Build history of the part. All positions in model axes, mm. Coordinates: 2 decimals unless noted, no trailing zeros. Order: outer loops, then holes, each group sorted by start corner. A loop starts at its lowest first (then second) coordinate and runs counter-clockwise, first axis right, second up. Notation, with made-up numbers: (60.5, 24.25) - (107.5, 24.25) arc R6 cw to (107.5, 35.25) - close; hole circle Ø9 at (73.25, 67). An arc over 180 degrees is marked (long way). One line per item, written item: value.
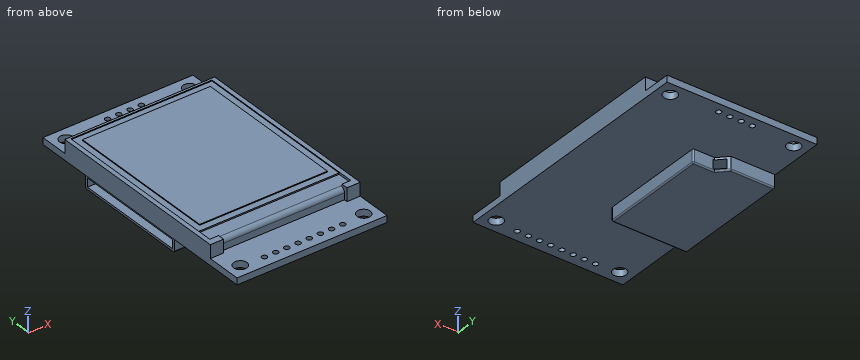
Autodesk Fusion 360 part; units mm, degrees
sketch "Sketch1" plane through (0, 0, 0) normal (0, 0, 1) x (1, 0, 0)
  line L0 (0, 0) -> (34, 0)
  line L1 (34, 0) -> (34, 58)
  line L2 (34, 58) -> (0, 58)
  line L3 (0, 58) -> (0, 0)
  circle A0 centre (3, 3) radius 1.5
  circle A1 centre (31, 3) radius 1.5
  circle A2 centre (3, 55) radius 1.5
  circle A3 centre (31, 55) radius 1.5
  dimension "d1" = 34
  dimension "d2" = 58
  dimension "d3" = 3
  dimension "d4" = 3
  dimension "d5" = 3
  dimension "d6" = 3
  dimension "d7" = 3
  dimension "d8" = 3
  dimension "d9" = 3
  dimension "d10" = 3
  dimension "d11" = 3
  dimension "d12" = 3
  dimension "d13" = 3
  dimension "d14" = 3
extrude "Extrude1" add sketch "Sketch1" along normal blind 1.5
sketch "Sketch2" plane through (0, 0, 1.5) normal (0, 0, 1) x (-1, 0, 0)
  circle A0 centre (-31, -3) radius 1.5
  circle A1 centre (-3, -55) radius 1.5
  circle A2 centre (-3, -3) radius 1.5
  circle A3 centre (-31, -55) radius 1.5
  line L0 (0, -58) -> (0, 0)
  line L1 (0, 0) -> (-34, 0)
  line L2 (-34, 0) -> (-34, -58)
  line L3 (-34, -58) -> (0, -58)
  line L4 (0, -8) -> (-34, -8)
  line L5 (-34, -8) -> (-34, -51.5)
  line L6 (-34, -51.5) -> (0, -51.5)
  line L7 (0, -51.5) -> (0, -8)
  dimension "d17" = 43.5
  dimension "d18" = 34
  dimension "d19" = 8
extrude "Extrude2" add sketch "Sketch2" along normal blind 3 contours L0 L2 L4 L5 L6 L7
sketch "Sketch3" plane through (0, 0, 4.5) normal (0, 0, 1) x (-1, 0, 0)
  line L0 (0, -51.5) -> (0, -8)
  line L1 (0, -8) -> (-34, -8)
  line L2 (-34, -8) -> (-34, -51.5)
  line L3 (-34, -51.5) -> (0, -51.5)
  line L4 (-1, -13) -> (-33, -13)
  line L5 (-33, -13) -> (-33, -51)
  line L6 (-33, -51) -> (-1, -51)
  line L7 (-1, -51) -> (-1, -13)
  line L8 (-3, -13) -> (-31, -13)
  line L9 (-31, -13) -> (-31, -8)
  line L10 (-31, -8) -> (-3, -8)
  line L11 (-3, -8) -> (-3, -13)
  line L12 (-3, -9.5) -> (-1, -9.5)
  line L13 (-1, -9.5) -> (-1, -13)
  line L14 (-1, -13) -> (-3, -13)
  line L15 (-3, -13) -> (-3, -9.5)
  line L16 (-31, -9.5) -> (-33, -9.5)
  line L17 (-33, -9.5) -> (-33, -13)
  line L18 (-33, -13) -> (-31, -13)
  line L19 (-31, -13) -> (-31, -9.5)
  dimension "d22" = 5
  dimension "d23" = 0.5
  dimension "d24" = 1
  dimension "d25" = 1
  dimension "d38" = 28
  dimension "d39" = 3
  dimension "d42" = 1.5
  dimension "d43" = 1.5
extrude "Extrude6" cut sketch "Sketch3" against normal blind 3 contours L4 L11 L12 L13 L14 L15 | L4 L9 L16 L17 L18 L19
extrude "Extrude5" cut sketch "Sketch3" against normal blind 3 contours L1 L4 L8 L9 L10 L11 L15 L19
sketch "Sketch4" plane through (0, 0, 1.5) normal (0, 0, 1) x (-1, 0, 0)
  line L0 (0, -58) -> (0, -51.5)
  line L1 (-34, -51.5) -> (-34, -58)
  circle A0 centre (-8.1, -2.5) radius 0.6
  circle A1 centre (-10.64, -2.5) radius 0.6
  circle A2 centre (-13.18, -2.5) radius 0.6
  circle A3 centre (-15.72, -2.5) radius 0.6
  circle A4 centre (-18.26, -2.5) radius 0.6
  circle A5 centre (-20.8, -2.5) radius 0.6
  circle A6 centre (-23.34, -2.5) radius 0.6
  circle A7 centre (-25.88, -2.5) radius 0.6
  line L2 (0, -51.5) -> (-34, -51.5)
  line L3 (-34, -58) -> (0, -58)
  circle A8 centre (-3, -55) radius 1.5
  circle A9 centre (-31, -55) radius 1.5
  dimension "d27" = 1.2
  dimension "d29" = 8.1
  dimension "d32" = -2.54
  dimension "d33" = 0
extrude "Extrude3" cut sketch "Sketch4" against normal blind 1.5 contours A0 | A1 | A2 | A3 | A4 | A5 | A6 | A7
extrude "Extrude4" cut sketch "Sketch3" against normal blind 0.1 contours L4 L5 L6 L7 L8 L14 L18
extrude "Extrude7" cut sketch "Sketch3" against normal blind 0.2 contours L4 L5 L6 L7 L8 L14 L18
sketch "Sketch5" plane through (0, 0, 4.3) normal (0, 0, 1) x (-1, 0, 0)
  line L0 (-33, -51) -> (-1, -51)
  line L1 (-1, -51) -> (-1, -13)
  line L2 (-1, -13) -> (-33, -13)
  line L3 (-33, -13) -> (-33, -51)
  line L4 (-2.5, -49.5) -> (-31.5, -49.5)
  line L5 (-31.5, -49.5) -> (-31.5, -14.5)
  line L6 (-31.5, -14.5) -> (-2.5, -14.5)
  line L7 (-2.5, -14.5) -> (-2.5, -49.5)
  dimension "d48" = 1.5
  dimension "d49" = 1.5
  dimension "d50" = 1.5
  dimension "d51" = 1.5
extrude "Extrude8" add sketch "Sketch5" along normal blind 0.2 contours L4 L5 L6 L7
sketch "Sketch6" plane through (0, 0, 1.5) normal (0, 0, 1) x (-1, 0, 0)
  line L0 (0, -51.5) -> (-34, -51.5)
  line L1 (-34, -51.5) -> (-34, -58)
  line L2 (-34, -58) -> (0, -58)
  line L3 (0, -58) -> (0, -51.5)
  circle A0 centre (-3, -55) radius 1.5
  circle A1 centre (-31, -55) radius 1.5
  circle A2 centre (-13, -55.8) radius 0.6
  circle A3 centre (-15.54, -55.8) radius 0.6
  circle A4 centre (-18.08, -55.8) radius 0.6
  circle A5 centre (-20.62, -55.8) radius 0.6
  dimension "d54" = 1.2
  dimension "d55" = 13
  dimension "d56" = 2.2
  dimension "d59" = -2.54
  dimension "d60" = 0
extrude "Extrude9" cut sketch "Sketch6" against normal blind 1.5 contours A2 | A3 | A4 | A5
sketch "Sketch7" plane through (0, 0, 1.5) normal (0, 0, 1) x (-1, 0, 0)
  circle A0 centre (-20.8, -2.5) radius 0.6
  circle A1 centre (-10.64, -2.5) radius 0.6
  circle A2 centre (-13.18, -2.5) radius 0.6
  circle A3 centre (-23.34, -2.5) radius 0.6
  circle A4 centre (-18.26, -2.5) radius 0.6
  circle A5 centre (-8.1, -2.5) radius 0.6
  circle A6 centre (-15.72, -2.5) radius 0.6
  circle A7 centre (-25.88, -2.5) radius 0.6
  circle A8 centre (-3, -3) radius 1.5
  circle A9 centre (-31, -3) radius 1.5
  line L0 (-31, -9.5) -> (-33, -9.5)
  line L1 (-33, -9.5) -> (-33, -13)
  line L2 (-33, -13) -> (-1, -13)
  line L3 (-1, -13) -> (-1, -9.5)
  line L4 (-1, -9.5) -> (-3, -9.5)
  line L5 (-3, -9.5) -> (-3, -8)
  line L6 (-3, -8) -> (0, -8)
  line L7 (0, -8) -> (0, 0)
  line L8 (0, 0) -> (-34, 0)
  line L9 (-34, 0) -> (-34, -8)
  line L10 (-34, -8) -> (-31, -8)
  line L11 (-31, -8) -> (-31, -9.5)
  line L12 (-1, -13) -> (-33, -13)
  line L13 (-33, -13) -> (-33, -9.5)
  line L14 (-33, -9.5) -> (-1, -9.5)
  line L15 (-1, -9.5) -> (-1, -13)
  line L16 (-3, -9.5) -> (-31, -9.5)
  line L17 (-31, -9.5) -> (-31, -8.75)
  line L18 (-31, -8.75) -> (-3, -8.75)
  line L19 (-3, -8.75) -> (-3, -9.5)
extrude "Extrude10" add sketch "Sketch7" along normal blind 2.5 contours L0 L1 L2 L3 L4 L12 L13 L14 L15 L16 | L5 L11 L14 L16 L17 L18 L19
fillet "Fillet2" radius 1 1 edges at (17, 8.75, 4)
sketch "Sketch8" plane through (0, 0, 0) normal (0, 0, -1) x (1, 0, 0)
  circle A0 centre (15.54, -55.8) radius 0.6
  circle A1 centre (18.08, -55.8) radius 0.6
  circle A2 centre (13, -55.8) radius 0.6
  circle A3 centre (20.62, -55.8) radius 0.6
  circle A4 centre (20.8, -2.5) radius 0.6
  circle A5 centre (10.64, -2.5) radius 0.6
  circle A6 centre (13.18, -2.5) radius 0.6
  circle A7 centre (23.34, -2.5) radius 0.6
  circle A8 centre (18.26, -2.5) radius 0.6
  circle A9 centre (8.1, -2.5) radius 0.6
  circle A10 centre (15.72, -2.5) radius 0.6
  circle A11 centre (25.88, -2.5) radius 0.6
  circle A12 centre (31, -3) radius 1.5
  circle A13 centre (3, -55) radius 1.5
  circle A14 centre (3, -3) radius 1.5
  circle A15 centre (31, -55) radius 1.5
  line L0 (0, 0) -> (0, -58)
  line L1 (0, -58) -> (34, -58)
  line L2 (34, -58) -> (34, 0)
  line L3 (34, 0) -> (0, 0)
  line L4 (0, -19) -> (17, -19)
  line L5 (10, -45.5) -> (0, -45.5)
  line L6 (0, -45.5) -> (0, -19)
  line L7 (10, -45.5) -> (12.1213, -43.3787)
  line L8 (12.1213, -43.3787) -> (17, -43.3787)
  line L9 (17, -43.3787) -> (17, -19)
  dimension "d66" = 19
  dimension "d68" = 26.5
  dimension "d69" = 10
  dimension "d70" = 3
  dimension "d71" = 135
extrude "Extrude11" add sketch "Sketch8" along normal blind 3 contours L0 L4 L5 L6 L7 L8 L9
sketch "Sketch9" plane through (0, 0, 0) normal (-1, 0, 0) x (0, -1, 0)
  line L0 (-58, 0) -> (-45.5, 0)
  line L1 (-45.5, 0) -> (-45.5, -3)
  line L2 (-45.5, -3) -> (-19, -3)
  line L3 (-19, -3) -> (-19, 0)
  line L4 (-19, 0) -> (0, 0)
  line L5 (0, 0) -> (0, 1.5)
  line L6 (0, 1.5) -> (-8, 1.5)
  line L7 (-8, 1.5) -> (-8, 4.5)
  line L8 (-8, 4.5) -> (-51.5, 4.5)
  line L9 (-51.5, 4.5) -> (-51.5, 1.5)
  line L10 (-51.5, 1.5) -> (-58, 1.5)
  line L11 (-58, 1.5) -> (-58, 0)
  line L12 (-45, -0.5) -> (-19.5, -0.5)
  line L13 (-19.5, -0.5) -> (-19.5, -2.5)
  line L14 (-19.5, -2.5) -> (-45, -2.5)
  line L15 (-45, -2.5) -> (-45, -0.5)
  dimension "d74" = 0.5
  dimension "d75" = 0.5
  dimension "d76" = 0.5
  dimension "d77" = 0.5
extrude "Extrude12" cut sketch "Sketch9" against normal blind 12.5 contours L12 L13 L14 L15
fillet "Fillet3" radius 0.3 8 edges at (5, 45.5, -3) (11.0607, 44.4393, -3) (14.5607, 43.3787, -3) (17, 31.1893, -3) (8.5, 19, -3) (17, 43.3787, -1.5) (10, 45.5, -1.5) (17, 19, -1.5)
sketch "Sketch10" plane through (0, 0, 0) normal (-1, 0, 0) x (0, -1, 0)
  arc A0 (-19.3, -3) -> (-19, -2.7) centre (-19.3, -2.7) ccw
  line L0 (-19, -2.7) -> (-19, 0)
  line L1 (-19, 0) -> (0, 0)
  line L2 (0, 0) -> (0, 1.5)
  line L3 (0, 1.5) -> (-8, 1.5)
  line L4 (-8, 1.5) -> (-8, 4.5)
  line L5 (-8, 4.5) -> (-51.5, 4.5)
  line L6 (-51.5, 4.5) -> (-51.5, 1.5)
  line L7 (-51.5, 1.5) -> (-58, 1.5)
  line L8 (-58, 1.5) -> (-58, 0)
  line L9 (-58, 0) -> (-45.5, 0)
  line L10 (-45.5, 0) -> (-45.5, -2.7)
  arc A1 (-45.5, -2.7) -> (-45.2, -3) centre (-45.2, -2.7) ccw
  line L11 (-45.2, -3) -> (-19.3, -3)
  line L12 (-19.5, -0.5) -> (-19.5, -2.5)
  line L13 (-19.5, -2.5) -> (-45, -2.5)
  line L14 (-45, -2.5) -> (-45, -0.5)
  line L15 (-45, -0.5) -> (-19.5, -0.5)
  line L16 (-45.5, 0) -> (-19, 0)
  line L17 (-19, 0) -> (-19, -3)
  line L18 (-19, -3) -> (-45.5, -3)
  line L19 (-45.5, -3) -> (-45.5, 0)
extrude "Extrude13" cut sketch "Sketch10" against normal blind 0.2 contours A0 L0 L10 A1 L11 L16 L17 L18 L19
1. Band-saw the part on B-B, the plane x = 23.34. Give the cut face in (y, z), and give its area (3 significant figures).
Values found:
outline: (0, 0) - (1.9, 0) - (1.9, 1.5) - (0, 1.5) - close; (3.1, 0) - (58, 0) - (58, 1.5) - (51.5, 1.5) - (51.5, 4.5) - (51, 4.5) - (51, 4.3) - (49.5, 4.3) - (49.5, 4.5) - (14.5, 4.5) - (14.5, 4.3) - (13, 4.3) - (13, 4) - (9.75, 4) arc R1 ccw to (8.75, 3) - (8.75, 1.5) - (3.1, 1.5) - close
area: 211 mm2
2. Flat gauge pins, fed straight in: P1, Ø2.5, axis at x = 31, y = 3, coming from the +Z side; P2, Ø10, axis at x = 21.5, y = 19.5, coming from the -Z side; P3, Ø2.5, axis at x = 11.5, y = 10.5, coming from the +Z side; P4, Ø1.4, axis at y = 36.5, z = -1, coming from the +X side. Where does each tip first touch, or does it go through?
Values found:
P1: passes through
P2: stops at z = -3
P3: stops at z = 4
P4: stops at x = 17
3. Probe line 1 along Y through (x, z) = (3, 0.7); line 2 along X through (y, z) = (8.5, 3.25); line 3 along Z through (x, y) = (15, 56.5). List the from-to ranges inside material, lowest first.
Values found:
line 1: y = 0 to 1.5, 4.5 to 53.5, 56.5 to 58
line 2: x = 0 to 3, 31 to 34
line 3: z = 0 to 1.5
4. Band-saw the part on C-C, the plane y = 55.8. Give the cut face in (x, z).
Values found:
outline: (0, 0) - (1.73, 0) - (1.73, 1.5) - (0, 1.5) - close; (4.27, 0) - (12.4, 0) - (12.4, 1.5) - (4.27, 1.5) - close; (13.6, 0) - (14.94, 0) - (14.94, 1.5) - (13.6, 1.5) - close; (16.14, 0) - (17.48, 0) - (17.48, 1.5) - (16.14, 1.5) - close; (18.68, 0) - (20.02, 0) - (20.02, 1.5) - (18.68, 1.5) - close; (21.22, 0) - (29.73, 0) - (29.73, 1.5) - (21.22, 1.5) - close; (32.27, 0) - (34, 0) - (34, 1.5) - (32.27, 1.5) - close
5. Band-saw the part on D-D, the plane x = 28. Give the cut face in (y, z), and give its area (3 significant figures).
Values found:
outline: (0, 0) - (58, 0) - (58, 1.5) - (51.5, 1.5) - (51.5, 4.5) - (51, 4.5) - (51, 4.3) - (49.5, 4.3) - (49.5, 4.5) - (14.5, 4.5) - (14.5, 4.3) - (13, 4.3) - (13, 4) - (9.75, 4) arc R1 ccw to (8.75, 3) - (8.75, 1.5) - (0, 1.5) - close
area: 212 mm2
6. Band-saw the part on A-A, the plane x = 8.1. Count the separate pieces of the cut face and the enclosed holes in it, and give its area (3 significant figures).
Values found:
separate pieces: 2
enclosed holes: 1
area: 239 mm2
